Source: three-view drawing plus pictorial views. Frame: mm from the lowest corner of the part. Give positions to 0.01 mm unless a question says otherwise; leave off trailing zeros. Order: outer loops, then holes, each group sorted by start corner. A loop starts at its lowest first (then second) coordinate and runs counter-clockwise, first axis right, second up. Notation, with made-up numbers: (27.25, 30.5) -> (67.25, 30.5) arc R8 cw to (67.25, 39.5) -> close; hole circle Ø1 at (82.5, 31.25). An arc over 180 degrees is marked (long way). Answer in a Markdown table with one row per item. Add a question column.
Q1. Cut plane B-B on z = 30.5. Return the cut outline in (x, y), and give its area (3 significant figures).
Q2. Line query: line 1 along Y through (x, z) = (1.55, 95); line 2 along Z through (x, y) = (3, 170); line 3 along Y through (x, z) = (1.6, 161). Output: solid intervals per line, ascending. Write a range as from..to.
Q3. Cut plane C-C on y = 76.5. Return the cut outline in (x, z), and give its area (3 significant figures).
Q4. Contact query for flat-ended pins moving along their axis: P1, Ø3, axis at y = 130, z = 95, coming from the -X side; P2, Ø2, axis at x = 1.5, y = 103, coming from the -Z side; P3, Ø1.2, axis at x = 3, z = 175.5, coming from the +Y side. Output: stop coordinate, or through.
Q5. Cut plane A-A on x = 1.45. Return the cut outline in (y, z), and give its area (3 significant figures).
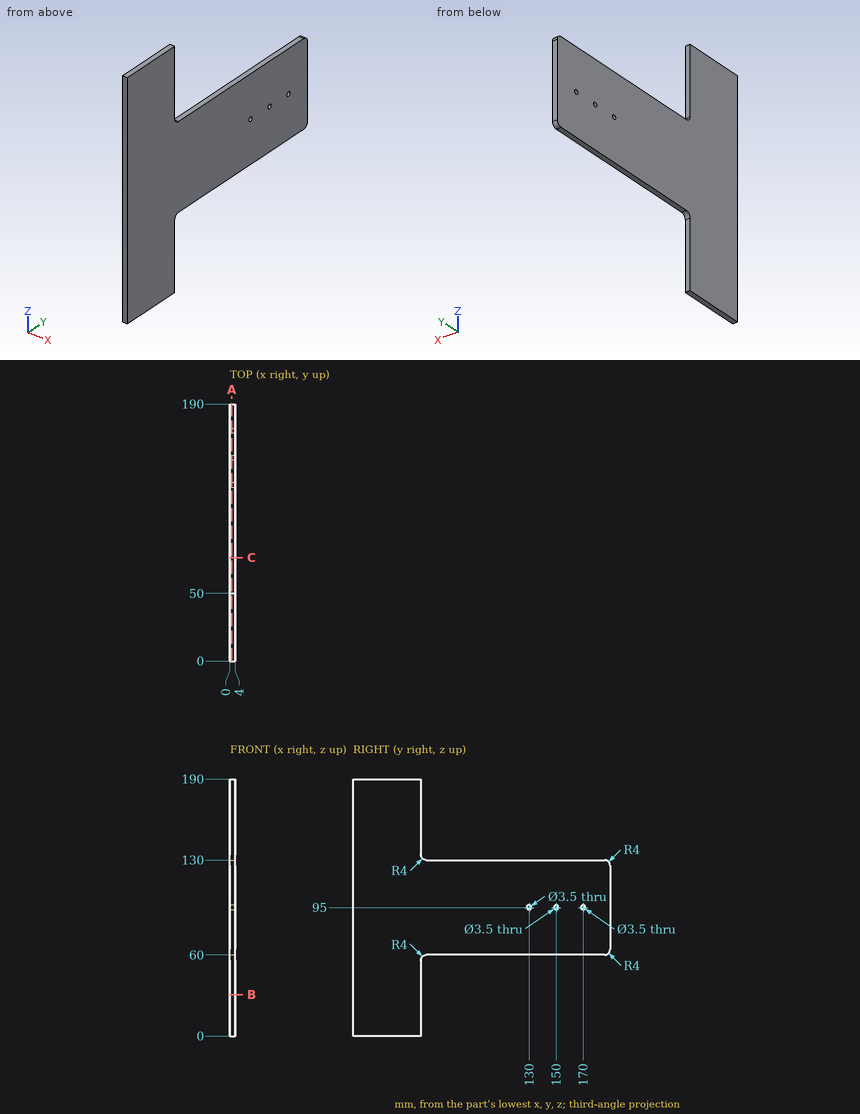
Completed:
| question | item | result |
|---|---|---|
| 1 | outline | (0, 0) -> (4, 0) -> (4, 50) -> (0, 50) -> close |
| 1 | area | 200 mm² |
| 2 | line 1 | y = 0..128.25, 131.75..148.25, 151.75..168.25, 171.75..190 |
| 2 | line 2 | z = 60..93.25, 96.75..130 |
| 2 | line 3 | y = 0..50 |
| 3 | outline | (0, 60) -> (4, 60) -> (4, 130) -> (0, 130) -> close |
| 3 | area | 280 mm² |
| 4 | P1 | passes through |
| 4 | P2 | stops at z = 60 |
| 4 | P3 | stops at y = 50 |
| 5 | outline | (0, 0) -> (50, 0) -> (50, 56) arc R4 cw to (54, 60) -> (186, 60) arc R4 ccw to (190, 64) -> (190, 126) arc R4 ccw to (186, 130) -> (54, 130) arc R4 cw to (50, 134) -> (50, 190) -> (0, 190) -> close; hole circle Ø3.5 at (130, 95); hole circle Ø3.5 at (150, 95); hole circle Ø3.5 at (170, 95) |
| 5 | area | 19,300 mm² |
